Verification items for the finished model (mm, model axes). Face numbers are marked on the shaded views. Round coordinates to 2 decimals unless told otherwise and drop trailing zeros. Loops run counter-clockwise (first coordinate to the right, second up) from the corner with the lowest first, then second, coordinate; pieces in that order, holes last. Notation, with made-up numbers: (76.25, -33.75) - (134.25, -33.75) arc R7 ccw to (134.25, -24.75) - close; hole circle Ø2 at (-28, -27). An arc over 180 degrees is marked (long way). Use a Markdown table: item, result. Add a question column.
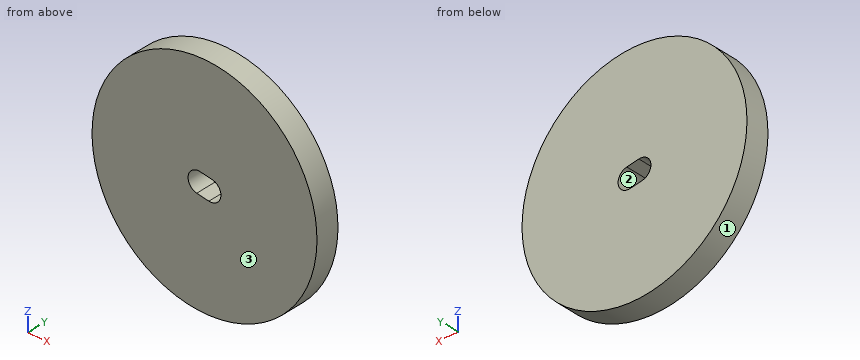
```python
from build123d import *

# Parameters (mm, degrees)
SKETCH_1_R          = 19
EXTRUDE_1_DEPTH     = 4
CUT_EXTRUDE_1_DEPTH = 28.166155414


with BuildPart() as part:
    # ｽｹｯﾁ1 → ﾎﾞｽ - 押し出し1 (new body)
    with BuildSketch(Plane(origin=(0, 0, 0), x_dir=(1, 0, 0), z_dir=(0, 1, 0))):
        with Locations(Location((0, 0, 0), (0, 0, 270))):
            Circle(SKETCH_1_R)
    extrude(amount=EXTRUDE_1_DEPTH)

    # ｽｹｯﾁ2 → ｶｯﾄ - 押し出し1 (cut, through all)
    with BuildSketch(Plane(origin=(0, 4, 0), x_dir=(1, 0, 0), z_dir=(0, 1, 0))):
        with BuildLine():
            Line((-1.306849725, 1.558759919), (0.739448512, 1.894941843))
            ThreePointArc((0.739448512, 1.894941843), (2.75, 0.451791569), (1.306849725, -1.558759919))
            Line((1.306849725, -1.558759919), (-0.739448512, -1.894941843))
            ThreePointArc((-0.739448512, -1.894941843), (-2.75, -0.451791569), (-1.306849725, 1.558759919))
        make_face()
    extrude(amount=-CUT_EXTRUDE_1_DEPTH, mode=Mode.SUBTRACT)


solid = part.part
```
Q1. Go/stop test with flat-tipped pins: pin 1 Ø2 at (y, z) = (2, 0.5) entering from +X; pin 2 Ø1.5 at (x, y) = (-3, 3) entering from -Z. Record where each tip stops, or that it passes through.
Q2. Section check B-B on x = 0. Record the cut outline in (y, z).
Q3. Section check D-D on z = -10. Record the cut outline in (x, y).
Q4. Thickness scan on line 1 along Z through (x, y) = (2, 2.7); line 2 along X through (y, z) = (3.15, -1); line 3 along X through (y, z) = (1.6, -11.5). Record the ranges inside material, lowest first.
Q5. Release check for a two-part mould opening along Z. For the marked faces 1, 2 and 3 record: +Z half, -Z half, draft (parallel to the pull), parting line (faces both ways), or undercut.
Q6. Section check C-C on y = 1.95. Record the cut outline in (x, z), plus the area to 3 significant figures.
Q7. Section check A-A on z = 0. Record the cut outline in (x, y), plus the area to 3 significant figures.
Determined:
| question | item | result |
|---|---|---|
| 1 | pin 1 | stops at x = 19 |
| 1 | pin 2 | stops at z = -18.87 |
| 2 | outline | (0, -19) - (4, -19) - (4, -1.77) - (0, -1.77) - close; (0, 1.77) - (4, 1.77) - (4, 19) - (0, 19) - close |
| 3 | outline | (-16.16, 0) - (16.16, 0) - (16.16, 4) - (-16.16, 4) - close |
| 4 | line 1 | z = -18.89 to -1.62, 1.28 to 18.89 |
| 4 | line 2 | x = -18.97 to -2.33, 2.56 to 18.97 |
| 4 | line 3 | x = -15.12 to 15.12 |
| 5 | face 1 | parting line |
| 5 | face 2 | undercut |
| 5 | face 3 | draft |
| 6 | outline | circle Ø38 at (0, 0); hole (-1.31, -1.56) - (0.74, -1.89) arc R1.75 ccw to (1.31, 1.56) - (-0.74, 1.89) arc R1.75 ccw to start |
| 6 | area | 1,120 mm² |
| 7 | outline | (-19, 0) - (-2.77, 0) - (-2.77, 4) - (-19, 4) - close; (2.77, 0) - (19, 0) - (19, 4) - (2.77, 4) - close |
| 7 | area | 130 mm² |
